```python
from build123d import *

# Parameters (mm, degrees)
SKETCH1_W           = 127
SKETCH1_H           = 76.2
SKETCH1_R           = 24.13
BOSS_EXTRUDE1_DEPTH = 5.08
CAVITY1_START       = -13.407959225
CAVITY1_OUTLINE_W   = 5.08
CAVITY1_OUTLINE_H   = 60.96
CAVITY1_DEPTH       = 5.08


# Read off the part's stored shape, not the designer's step: Cavity1
with BuildPart() as part:
    # Sketch1 → Boss-Extrude1 (new body)
    with BuildSketch(Plane(origin=(0, 0, 0), x_dir=(1, 0, 0), z_dir=(0, 1, 0))):
        Rectangle(SKETCH1_W, SKETCH1_H)
        with Locations(Location((-33.925370199, 0, 0), (0, 0, 270))):
            Circle(SKETCH1_R, mode=Mode.SUBTRACT)
    extrude(amount=BOSS_EXTRUDE1_DEPTH)

    # Cavity1 outline → Cavity1 (cut)
    with BuildSketch(Plane.YZ.offset(CAVITY1_START)):
        with Locations((2.54, -1.5875)):
            Rectangle(CAVITY1_OUTLINE_W, CAVITY1_OUTLINE_H)
    extrude(amount=CAVITY1_DEPTH, mode=Mode.SUBTRACT)


solid = part.part
```
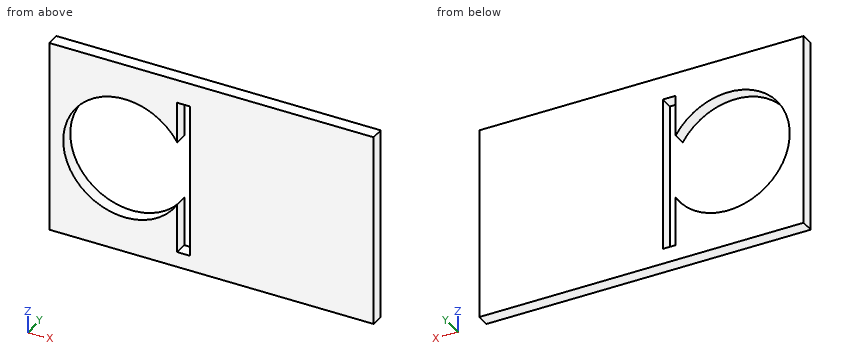
Here's how the part is built. I have some questions about the finished solid (model axes, mm). Round coordinates to 2 decimals unless told otherwise and drop trailing zeros. Write each loop counter-clockwise with the first axis right and the second up, starting at its lowest first coordinate (ties: lowest second). Pieces come first, ordered by that corner, then holes.
Q1. Please list where these lines run through material, in increasing order: probe 1 along X at (y, z) = (2.35, 0); probe 2 along X at (y, z) = (1.1, 13); probe 3 along X at (y, z) = (1.55, 26).
Q2. If we section it at A-A on z = 0: Write out the boundary of the cut face in (x, y), plus the area to 3 significant figures.
Q3. If we section it at C-C on z = 22: Write out the boundary of the cut face in (x, y), plus the area to 3 significant figures.
Q4. If we section it at B-B on y = 1: Write out the boundary of the cut face in (x, z), plus the area to 3 significant figures.
Answer below:
1. probe 1: x = -63.5 to -58.06, -8.33 to 63.5
1. probe 2: x = -63.5 to -54.25, -13.6 to -13.41, -8.33 to 63.5
1. probe 3: x = -63.5 to -13.41, -8.33 to 63.5
2. outline: (-63.5, 0) - (-58.06, 0) - (-58.06, 5.08) - (-63.5, 5.08) - close; (-8.33, 0) - (63.5, 0) - (63.5, 5.08) - (-8.33, 5.08) - close
2. area: 393 mm2
3. outline: (-63.5, 0) - (-43.84, 0) - (-43.84, 5.08) - (-63.5, 5.08) - close; (-24.01, 0) - (-13.41, 0) - (-13.41, 5.08) - (-24.01, 5.08) - close; (-8.33, 0) - (63.5, 0) - (63.5, 5.08) - (-8.33, 5.08) - close
3. area: 519 mm2
4. outline: (-63.5, -38.1) - (63.5, -38.1) - (63.5, 38.1) - (-63.5, 38.1) - close; hole (-13.41, -32.07) - (-8.33, -32.07) - (-8.33, 28.89) - (-13.41, 28.89) - (-13.41, 12.7) arc R24.13 ccw (long way) to (-13.41, -12.7) - close
4. area: 7,600 mm2
